Source: CAD feature listing. Evaluate the final solid. Frame: model axes, mm. A direction names the side the tool comes from. Round coordinates to 2 decimals unless told otherwise and drop trailing zeros. Loops run counter-clockwise (first coordinate to the right, second up) from the corner with the lowest first, then second, coordinate; pieces in that order, holes last. Notation, with made-up numbers: M -18.5,1.25 L 16.5,1.25 A34 cw 16.5,37.25 Z; hole C 25.25,83 d6. An arc over 180 degrees is marked long. Write each question's results on one line, items separated by ' | '. Start each with the question number.
1. Section B-B on z = 2.75. Output: boundary loops of the cut face in (x, y), and give its area (3 significant figures).
2. Ray query, line 1 (Y direction, x = 4.75, z = -0.5); line 2 (Z direction, x = -3.25, y = -0.75); line 3 (X direction, y = 0, z = -0.9). Return the intervals inside material, ascending.
3. Section A-A on z = 0.75. Output: boundary loops of the cut face in (x, y).
4. Contact query for flat-ended pins moving along their axis: pin 1 Ø3 at (x, z) = (-5, 1) entering from -Y; pin 2 Ø4.5 at (x, y) = (-2, -2) entering from -Z; pin 3 Ø1.5 at (x, z) = (4, 2.5) entering from +Y. Output: stop coordinate, or through.
5. Set-up query: faces 4 (the flat face through (-6, -2, -2.2)), 5 (the flat face through (2.5, 0.1, 3.5)). Return all of +Z, -Z, +X, -X, +Y, -Y with unobstructed straight access to the full face (end or side cutting, diameter ignored); none if empty.
6. Draft query along Y for faces 1 (the flat face through (-2, 2, 5)), 2 (the conical face through (6.94, 2.19, 2.91)), 3 (the cylindrical face through (-0.29, 2.23, 4.26)). Return one class per face: released by +Y, released by -Y, zero draft, split by the parting line, or undercut.
from build123d import *

# Parameters (mm, degrees)
SKETCH1_R           = 7.43
BOSS_EXTRUDE3_DEPTH = 5
BOSS_EXTRUDE3_TAPER = 3
SHELL1_T            = -1.5
SKETCH3_R           = 6.93
SKETCH3_R_2         = 5.927941481
BOSS_EXTRUDE4_DEPTH = 2.2
CUT_SWEEP1_PITCH    = 0.5
CHAMFER1_SIZE       = 0.3
CHAMFER1_SIZE_2     = 0.317026351
SKETCH7_R           = 2.25
CUT_EXTRUDE1_DEPTH  = 6


with BuildPart() as part:
    # Sketch1 → Boss-Extrude3 (new body)
    with BuildSketch(Plane.XY):
        Circle(SKETCH1_R)
    extrude(amount=BOSS_EXTRUDE3_DEPTH, taper=BOSS_EXTRUDE3_TAPER)

    # Shell1
    shell1_openings = [part.faces().sort_by_distance(p)[0] for p in [
        (0, 0, 0),
    ]]
    offset(amount=SHELL1_T, openings=shell1_openings, kind=Kind.INTERSECTION)


with BuildPart() as body_2:
    # Sketch3 → Boss-Extrude4 (new body)
    with BuildSketch(Plane(origin=(0, 0, 0), x_dir=(-1, 0, 0), z_dir=(0, 0, -1))):
        Circle(SKETCH3_R)
        Circle(SKETCH3_R_2, mode=Mode.SUBTRACT)
    extrude(amount=BOSS_EXTRUDE4_DEPTH)


with BuildPart() as part_1:
    add(part.part)

    # Combine1: union body 2
    add(body_2.part)

    # Cut-Sweep1: arcs per turn and ends read off the stored shape
    # Cut-Sweep1: the profile of Sketch6 screwed along a right-hand helix through 5 turns, 6 arcs to a turn; built about Z, then put on its axis
    cut_sweep1_z = Axis((0, 0, 0), (0, 0, 1))
    cut_sweep1_corners = [(6.527962418, -2.7236e-05, -0.497628173), (6.94947392, -0.002896154, -0.24778858), (6.955099869, 0.002729794, -0.737723981)]
    with BuildLine(mode=Mode.PRIVATE) as cut_sweep1_profile:
        Line(cut_sweep1_corners[0], cut_sweep1_corners[1])
        Line(cut_sweep1_corners[1], cut_sweep1_corners[2])
        Line(cut_sweep1_corners[2], cut_sweep1_corners[0])
    cut_sweep1_cap = Face(cut_sweep1_profile.wire())
    cut_sweep1_turn_angles = [0, 30, 60, 90, 120, 150, 180, 210, 240, 270, 300, 330, 360]
    cut_sweep1_turn_weights = [1, 0.8660254037844387, 1, 0.8660254037844387, 1, 0.8660254037844387, 1, 0.8660254037844387, 1, 0.8660254037844387, 1, 0.8660254037844387, 1]
    cut_sweep1_turn_rails = [Edge.make_bspline([Vector(p[0], p[1], 0).rotate(cut_sweep1_z, cut_sweep1_turn_angles[k]) / cut_sweep1_turn_weights[k] + Vector(0, 0, p[2] + CUT_SWEEP1_PITCH * cut_sweep1_turn_angles[k] / 360) for k in range(13)], [0, 0, 0, 1, 1, 2, 2, 3, 3, 4, 4, 5, 5, 6, 6, 6], 2, cut_sweep1_turn_weights) for p in cut_sweep1_corners]
    cut_sweep1_turn_sides = [Face.make_surface_from_curves(cut_sweep1_turn_rails[p[0]], cut_sweep1_turn_rails[p[1]]) for p in [(0, 1), (1, 2), (2, 0)]]
    cut_sweep1 = Plane(origin=(0, 0, -2.2), x_dir=(0.7071067811865512, 0.7071067811865438, 0), z_dir=(0, 0, 1)) * Solid(Shell([*[p.moved(Location((0, 0, CUT_SWEEP1_PITCH * i))) for i in range(5) for p in cut_sweep1_turn_sides], cut_sweep1_cap, cut_sweep1_cap.rotate(cut_sweep1_z, 1800).moved(Location((0, 0, CUT_SWEEP1_PITCH * 1800 / 360)))]))
    add(cut_sweep1, mode=Mode.SUBTRACT)

    # Chamfer1
    # the kernel refuses this chamfer: 0.317026351, 0.3 mm, written as the material it takes off along each edge
    with BuildSketch(Plane(origin=(0, 0, 5), x_dir=(1, 0, 0), z_dir=(0, 1, 0))) as chamfer1_piece_1:
        Polygon((7.167961104 + CHAMFER1_SIZE * 0.0523359562429, CHAMFER1_SIZE * 0.998629534755), (7.167961104 - CHAMFER1_SIZE_2, 0), (7.167961104, 0), align=None)
    revolve(axis=Axis((0, 0, 5), (0, 0, -1)), mode=Mode.SUBTRACT)

    # Sketch7 → Cut-Extrude1 (cut)
    with BuildSketch(Plane.XY.offset(5)):
        Circle(SKETCH7_R)
    extrude(amount=-CUT_EXTRUDE1_DEPTH, mode=Mode.SUBTRACT)


solid = part_1.part
Taken from the geometry:
1) outline: C 0,0 d14.57; hole C 0,0 d11.57 | area: 61.7 mm^2
2) line 1: -4.92 to -3.55, 3.55 to 4.95 | line 2: 3.5 to 5 | line 3: -6.71 to -5.93, 5.93 to 6.78
3) outline: C 0,0 d14.78; hole C 0,0 d11.78
4) pin 1: y = -6.5 | pin 2: z = 3.5 | pin 3: y = 6.54
5) face 4: -Z, +X, -X, +Y, -Y | face 5: -Z
6) face 1: zero draft | face 2: split by the parting line | face 3: undercut
